Could you check a few things on this model? Use its own coordinates, in mm. Face numbers are marked on the shaded views. A direction names the side the tool comes from. Coordinates: 2 decimals unless noted, no trailing zeros. Loops run counter-clockwise (first coordinate to the right, second up) from the corner with the lowest first, then second, coordinate; pieces in that order, holes last.
from build123d import *

# Parameters (mm, degrees)
SKETCH1_R           = 3
BOSS_EXTRUDE1_DEPTH = 4
BOSS_EXTRUDE2_DEPTH = 3
SKETCH3_R           = 3
BOSS_EXTRUDE3_DEPTH = 4
FILLET2_R           = 35
CHAMFER1_SIZE       = 1
CHAMFER2_SIZE       = 1


with BuildPart() as part:
    # Sketch1 → Boss-Extrude1 (new body)
    with BuildSketch(Plane(origin=(0, 0, 0), x_dir=(1, 0, 0), z_dir=(0, 1, 0))):
        with Locations(Location((0, 0, 0), (0, 0, 270))):
            Circle(SKETCH1_R)
    extrude(amount=-BOSS_EXTRUDE1_DEPTH)

    # Sketch2 → Boss-Extrude2 (add)
    with BuildSketch(Plane(origin=(0, 0, 0), x_dir=(1, 0, 0), z_dir=(0, 1, 0))):
        Polygon((-3.25, 43), (-3.25, 13.856601718), (-13.856601718, 3.25), (-43, 3.25), (-43, -3.25), (-13.856601718, -3.25), (-3.25, -13.856601718), (-3.25, -43), (3.25, -43), (3.25, -13.856601718), (13.856601718, -3.25), (43, -3.25), (43, 3.25), (13.856601718, 3.25), (3.25, 13.856601718), (3.25, 43), align=None)
    extrude(amount=BOSS_EXTRUDE2_DEPTH)

    # Sketch3 → Boss-Extrude3 (add)
    with BuildSketch(Plane(origin=(0, 3, 0), x_dir=(1, 0, 0), z_dir=(0, 1, 0))):
        with Locations(Location((-37.5, 0, 0), (0, 0, 270))):
            Circle(SKETCH3_R)
        with Locations(Location((0, 37.5, 0), (0, 0, 270))):
            Circle(SKETCH3_R)
        with Locations(Location((37.5, 0, 0), (0, 0, 270))):
            Circle(SKETCH3_R)
        with Locations(Location((0, -37.5, 0), (0, 0, 270))):
            Circle(SKETCH3_R)
    extrude(amount=BOSS_EXTRUDE3_DEPTH)

    # Fillet2
    # the kernel refuses this fillet: 35 mm, written as the material it adds along each edge
    with BuildSketch(Plane(origin=(-13.856601718, 0, -3.25), x_dir=(0.7071067811865472, 0, -0.7071067811865478), z_dir=(0, 1, 0)), Plane(origin=(-3.25, 0, -13.856601718), x_dir=(0, 0, -1), z_dir=(0, 1, 0)), Plane(origin=(-13.856601718, 0, 3.25), x_dir=(-1, 0, 0), z_dir=(0, 1, 0)), Plane(origin=(-3.25, 0, 13.856601718), x_dir=(-0.7071067811865476, 0, -0.7071067811865475), z_dir=(0, 1, 0))) as fillet2_piece_1:
        with BuildLine():
            CenterArc((FILLET2_R * 0.414213562373, FILLET2_R), FILLET2_R, 225, 45)
            Line((-FILLET2_R * 0.292893218813, FILLET2_R * 0.292893218813), (0, 0))
            Line((0, 0), (FILLET2_R * 0.414213562373, 0))
        make_face()
    extrude(amount=3)
    with BuildSketch(Plane(origin=(3.25, 0, -13.856601718), x_dir=(0, 0, -1), z_dir=(0, 1, 0)), Plane(origin=(13.856601718, 0, -3.25), x_dir=(-0.7071067811865475, 0, -0.7071067811865476), z_dir=(0, 1, 0)), Plane(origin=(13.856601718, 0, 3.25), x_dir=(1, 0, 0), z_dir=(0, 1, 0)), Plane(origin=(3.25, 0, 13.856601718), x_dir=(0.7071067811865477, 0, -0.7071067811865474), z_dir=(0, 1, 0))) as fillet2_piece_2:
        with BuildLine():
            CenterArc((FILLET2_R * 0.414213562373, -FILLET2_R), FILLET2_R, 90, 45)
            Line((-FILLET2_R * 0.292893218813, -FILLET2_R * 0.292893218813), (0, 0))
            Line((0, 0), (FILLET2_R * 0.414213562373, 0))
        make_face()
    extrude(amount=3)

    # Chamfer1
    # the kernel refuses this chamfer: 1 mm, written as the material it adds along each edge
    with BuildSketch(Plane(origin=(-37.5, 3, 0), x_dir=(0, 0, 1), z_dir=(-1, 0, 0))) as chamfer1_piece_1_section:
        Polygon((3 + CHAMFER1_SIZE, 0), (3, CHAMFER1_SIZE), (3, 0), align=None)
    chamfer1_piece_1 = revolve(axis=Axis((-37.5, 3, 0), (0, 1, 0)), mode=Mode.PRIVATE)
    chamfer1_piece_1 = split(chamfer1_piece_1, bisect_by=Plane(origin=(-34.177083345, 3.132594622, 3.25), z_dir=(0, 0, -1)), keep=Keep.TOP, mode=Mode.PRIVATE)
    chamfer1_piece_1 = split(chamfer1_piece_1, bisect_by=Plane(origin=(-34.177083345, 3.132594622, -3.25), z_dir=(0, 0, 1)), keep=Keep.TOP, mode=Mode.PRIVATE)
    add(chamfer1_piece_1)
    with BuildSketch(Plane(origin=(0, 3, -37.5), x_dir=(0, 0, 1), z_dir=(-1, 0, 0))) as chamfer1_piece_2_section:
        Polygon((3 + CHAMFER1_SIZE, 0), (3, CHAMFER1_SIZE), (3, 0), align=None)
    chamfer1_piece_2 = revolve(axis=Axis((0, 3, -37.5), (0, 1, 0)), mode=Mode.PRIVATE)
    chamfer1_piece_2 = split(chamfer1_piece_2, bisect_by=Plane(origin=(-3.25, 3.484784137, -40.984784137), z_dir=(1, 0, 0)), keep=Keep.TOP, mode=Mode.PRIVATE)
    chamfer1_piece_2 = split(chamfer1_piece_2, bisect_by=Plane(origin=(3.25, 3.484784137, -40.984784137), z_dir=(-1, 0, 0)), keep=Keep.TOP, mode=Mode.PRIVATE)
    add(chamfer1_piece_2)
    with BuildSketch(Plane(origin=(37.5, 3, 0), x_dir=(0, 0, 1), z_dir=(-1, 0, 0))) as chamfer1_piece_3_section:
        Polygon((3 + CHAMFER1_SIZE, 0), (3, CHAMFER1_SIZE), (3, 0), align=None)
    chamfer1_piece_3 = revolve(axis=Axis((37.5, 3, 0), (0, 1, 0)), mode=Mode.PRIVATE)
    chamfer1_piece_3 = split(chamfer1_piece_3, bisect_by=Plane(origin=(40.822916655, 3.132594622, -3.25), z_dir=(0, 0, 1)), keep=Keep.TOP, mode=Mode.PRIVATE)
    chamfer1_piece_3 = split(chamfer1_piece_3, bisect_by=Plane(origin=(40.822916655, 3.132594622, 3.25), z_dir=(0, 0, -1)), keep=Keep.TOP, mode=Mode.PRIVATE)
    add(chamfer1_piece_3)
    with BuildSketch(Plane(origin=(0, 3, 37.5), x_dir=(0, 0, 1), z_dir=(-1, 0, 0))) as chamfer1_piece_4_section:
        Polygon((3 + CHAMFER1_SIZE, 0), (3, CHAMFER1_SIZE), (3, 0), align=None)
    chamfer1_piece_4 = revolve(axis=Axis((0, 3, 37.5), (0, 1, 0)), mode=Mode.PRIVATE)
    chamfer1_piece_4 = split(chamfer1_piece_4, bisect_by=Plane(origin=(3.25, 3.484784137, 34.015215863), z_dir=(-1, 0, 0)), keep=Keep.TOP, mode=Mode.PRIVATE)
    chamfer1_piece_4 = split(chamfer1_piece_4, bisect_by=Plane(origin=(-3.25, 3.484784137, 34.015215863), z_dir=(1, 0, 0)), keep=Keep.TOP, mode=Mode.PRIVATE)
    add(chamfer1_piece_4)

    # Chamfer2
    chamfer2_edges = [part.edges().sort_by_distance(p)[0] for p in [
        (-3.25, 0, 35.6770382),
        (3.25, 0, 35.6770382),
        (0, 0, 43),
        (3.25, 0, -35.6770382),
        (-3.25, 0, -35.6770382),
        (-4.732121832, 0, -18.276782958),
        (-18.276782958, 0, -4.732121832),
        (-35.6770382, 0, -3.25),
        (-35.6770382, 0, 3.25),
        (-18.276782958, 0, 4.732121832),
        (-4.732121832, 0, 18.276782958),
        (4.732121832, 0, 18.276782958),
        (18.276782958, 0, 4.732121832),
        (35.6770382, 0, 3.25),
        (35.6770382, 0, -3.25),
        (18.276782958, 0, -4.732121832),
        (4.732121832, 0, -18.276782958),
        (43, 0, 0),
        (-43, 0, 0),
        (0, 0, -43),
    ]]
    chamfer(chamfer2_edges, length=CHAMFER2_SIZE)


solid = part.part
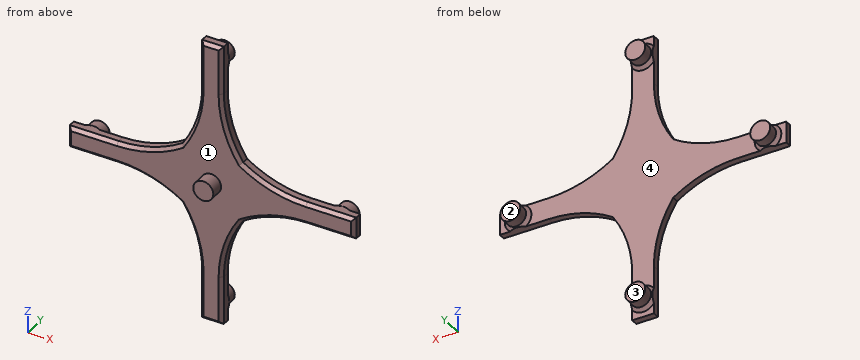
(1) I need wall thicknesses on probe 1 along X at (y, z) = (5.5, -37.5); probe 2 along Z at (x, y) = (35.5, 5.25); probe 3 along X at (y, z) = (1.5, 34.5). Which ranges of each line are inside material? Lowest first, please.
Answers:
probe 1: x = -3 to 3
probe 2: z = -2.24 to 2.24
probe 3: x = -3.25 to 3.25
(2) Imagine slicing it at A-A, the plane z = 0. Write out the boundary of the cut face in (x, y).
Answers:
outline: (-43, 1) - (-42, 0) - (-3, 0) - (-3, -4) - (3, -4) - (3, 0) - (42, 0) - (43, 1) - (43, 3) - (41.5, 3) - (40.5, 4) - (40.5, 7) - (34.5, 7) - (34.5, 4) - (33.5, 3) - (-33.5, 3) - (-34.5, 4) - (-34.5, 7) - (-40.5, 7) - (-40.5, 4) - (-41.5, 3) - (-43, 3) - close
(3) For pin 1 (0.8 mm diameter, centred on y = 2.5, z = -33, fed in from +X); pin 2 (0.8 mm diameter, centred on y = 3, z = -36.5, fed in from -X); pin 3 (21 mm diameter, centred on x = 8.5, z = 17, fed in from +Y); pin 4 (3.5 mm diameter, centred on x = 42, z = 0.5, fed in from +Y), each with a flat end and sliding along its axis, tell me the tip position at first contact or that it passes through.
Answers:
pin 1: stops at x = 3.25
pin 2: stops at x = -3.25
pin 3: stops at y = 3
pin 4: stops at y = 7
(4) Imagine slicing it at C-C, the plane z = 37.5. Write out the boundary of the cut face in (x, y).
Answers:
outline: (-3.25, 1) - (-2.25, 0) - (2.25, 0) - (3.25, 1) - (3.25, 3.75) - (3, 4) - (3, 7) - (-3, 7) - (-3, 4) - (-3.25, 3.75) - close
(5) Imagine slicing it at B-B, the plane y = 2. Write out the boundary of the cut face in (x, z), and give its area (3 significant figures).
Answers:
outline: (-43, -3.25) - (-28.35, -3.25) arc R35 cw to (-9.05, -9.05) arc R35 cw to (-3.25, -28.35) - (-3.25, -43) - (3.25, -43) - (3.25, -28.35) arc R35 cw to (9.05, -9.05) arc R35 cw to (28.35, -3.25) - (43, -3.25) - (43, 3.25) - (28.35, 3.25) arc R35 cw to (9.05, 9.05) arc R35 cw to (3.25, 28.35) - (3.25, 43) - (-3.25, 43) - (-3.25, 28.35) arc R35 cw to (-9.05, 9.05) arc R35 cw to (-28.35, 3.25) - (-43, 3.25) - close
area: 1,500 mm2
(6) We'd pull the mould along Z, two halves only. Please class the marked faces 3 and 4: +Z half, -Z half, draft (parallel to the pull), parting line (faces both ways), or undercut.
Answers:
face 3: draft
face 4: undercut
(7) Which directions (+Z, -Z, +X, -X, +Y, -Y) give clear straight access to the entire face, cutting with the end or side of a thin tool? Please do the marked faces 1 and 2.
Answers:
face 1: -Y
face 2: +Z, -Z, +X, -X, +Y
